from build123d import *

# Parameters (mm, degrees)
EXTRUDE_1_DEPTH = 4
FILLET_1_R      = 1
FILLET_2_R      = 1.3


with BuildPart() as part:
    # 草图1 → 凸台-拉伸1 (new body)
    with BuildSketch(Plane.XY):
        Polygon((0, 0), (0, -4), (-1.35, -4), (-1.35, -6.6), (0, -6.6), (0, -8.6), (3, -8.6), (3, -6.6), (4.35, -6.6), (4.35, -4), (3, -4), (3, 0), (30.5, 0), (30.5, 5), (38.5, 5), (38.5, 0), (66, 0), (66, -4), (64.65, -4), (64.65, -6.6), (66, -6.6), (66, -8.6), (69, -8.6), (69, -6.6), (70.35, -6.6), (70.35, -4), (69, -4), (69, 0), (96.5, 0), (96.5, 5), (104.5, 5), (104.5, 0), (132, 0), (143.5, 0), (143.5, -63), (148.5, -63), (148.5, -71), (143.5, -71), (143.5, -98.5), (139.5, -98.5), (139.5, -97.15), (136.9, -97.15), (136.9, -98.5), (134.9, -98.5), (134.9, -101.5), (136.9, -101.5), (136.9, -102.85), (139.5, -102.85), (139.5, -101.5), (143.5, -101.5), (143.5, -129), (148.5, -129), (148.5, -137), (143.5, -137), (143.5, -200), (132, -200), (104.5, -200), (104.5, -205), (96.5, -205), (96.5, -200), (69, -200), (69, -196), (70.35, -196), (70.35, -193.4), (69, -193.4), (69, -191.4), (66, -191.4), (66, -193.4), (64.65, -193.4), (64.65, -196), (66, -196), (66, -200), (38.5, -200), (38.5, -205), (30.5, -205), (30.5, -200), (3, -200), (3, -196), (4.35, -196), (4.35, -193.4), (3, -193.4), (3, -191.4), (0, -191.4), (0, -193.4), (-1.35, -193.4), (-1.35, -196), (0, -196), (0, -200), (-27.5, -200), (-27.5, -205), (-35.5, -205), (-35.5, -200), (-63, -200), (-63, -196), (-61.65, -196), (-61.65, -193.4), (-63, -193.4), (-63, -191.4), (-66, -191.4), (-66, -193.4), (-67.35, -193.4), (-67.35, -196), (-66, -196), (-66, -200), (-93.5, -200), (-93.5, -205), (-101.5, -205), (-101.5, -200), (-129, -200), (-140.5, -200), (-140.5, -137), (-145.5, -137), (-145.5, -129), (-140.5, -129), (-140.5, -101.5), (-136.5, -101.5), (-136.5, -102.85), (-133.9, -102.85), (-133.9, -101.5), (-131.9, -101.5), (-131.9, -98.5), (-133.9, -98.5), (-133.9, -97.15), (-136.5, -97.15), (-136.5, -98.5), (-140.5, -98.5), (-140.5, -71), (-145.5, -71), (-145.5, -63), (-140.5, -63), (-140.5, 0), (-129, 0), (-101.5, 0), (-101.5, 5), (-93.5, 5), (-93.5, 0), (-66, 0), (-66, -4), (-67.35, -4), (-67.35, -6.6), (-66, -6.6), (-66, -8.6), (-63, -8.6), (-63, -6.6), (-61.65, -6.6), (-61.65, -4), (-63, -4), (-63, 0), (-35.5, 0), (-35.5, 5), (-27.5, 5), (-27.5, 0), align=None)
    extrude(amount=EXTRUDE_1_DEPTH)

    # 圆角1
    fillet_1_edges = [part.edges().sort_by_distance(p)[0] for p in [
        (-145.5, -63, 2),
        (-145.5, -71, 2),
        (-145.5, -129, 2),
        (-145.5, -137, 2),
    ]]
    fillet(fillet_1_edges, radius=FILLET_1_R)

    # 圆角2
    fillet_2_edges = [part.edges().sort_by_distance(p)[0] for p in [
        (38.5, 5, 2),
        (30.5, 5, 2),
        (-27.5, 5, 2),
        (-35.5, 5, 2),
        (-93.5, 5, 2),
        (-101.5, 5, 2),
        (-101.5, -205, 2),
        (-93.5, -205, 2),
        (-35.5, -205, 2),
        (-27.5, -205, 2),
        (30.5, -205, 2),
        (38.5, -205, 2),
        (96.5, -205, 2),
        (104.5, -205, 2),
        (148.5, -137, 2),
        (148.5, -129, 2),
        (148.5, -71, 2),
        (148.5, -63, 2),
        (104.5, 5, 2),
        (96.5, 5, 2),
    ]]
    fillet(fillet_2_edges, radius=FILLET_2_R)


solid = part.part
For this review, take the finished solid that the model builds, in its own axes (mm). Give positions to 0.01 mm unless a question says otherwise; leave off trailing zeros. Loops run counter-clockwise (first coordinate to the right, second up) from the corner with the lowest first, then second, coordinate; pieces in that order, holes last. Notation, with made-up numbers: M 0,74.25 L 40,74.25 A14 cw 40,92.25 Z; hole C 10.25,32.5 d5. An arc over 180 degrees is marked long. Answer as a JSON object with one key per item and string values. Group by question number.
Q1. For probe 1 along Y at (x, z) = (-67, 0.7); probe 2 along Y at (x, z) = (37.5, 0.65); probe 3 along Y at (x, z) = (-68.5, 2.8), list the stretches that pass through material, from the lowest coordinate up. Write a range as [from, to].
Q2. Add section B-B on x = 44. Give the boundary of the cut face in (y, z).
Q3. Add section A-A on y = -142. Give the boundary of the cut face in (x, z).
Q4. Insertion check: P1, Ø1.8, axis at y = 1, z = 1.5, coming from the -X side; P2, Ø1.5, axis at x = 65.5, z = 2, coming from the -Y side; P3, Ø1.6, axis at y = -8, z = 1, coming from the -X side. Each pin has a flat end and moves straight along its axis. Give the tip position at first contact, or say it passes through.
Checked values:
{
 "1": {"probe 1": "[-200, -196], [-193.4, -6.6], [-4, 0]", "probe 2": "[-204.96, 4.96]", "probe 3": "[-200, 0]"},
 "2": {"outline": "M -200,0 L 0,0 L 0,4 L -200,4 Z"},
 "3": {"outline": "M -140.5,0 L 143.5,0 L 143.5,4 L -140.5,4 Z"},
 "4": {"P1": "x = -101.5", "P2": "y = -200", "P3": "x = -140.5"}
}
